The drawing under review shows one solid part. Ordinate dimensions are in mm from its lowest x, y, z. Coordinates: 2 decimals unless noted, no trailing zeros. Write each loop counter-clockwise with the first axis right and the second up, starting at its lowest first coordinate (ties: lowest second). Pieces come first, ordered by that corner, then holes. Notation, with made-up numbers: M 83.25,30.5 L 106.25,30.5 A17 ccw 106.25,50.5 Z; hole C 32,-5 d2. An arc over 180 degrees is marked long. Write each question's results on one line, items separated by ' | '. Start each with the question number.
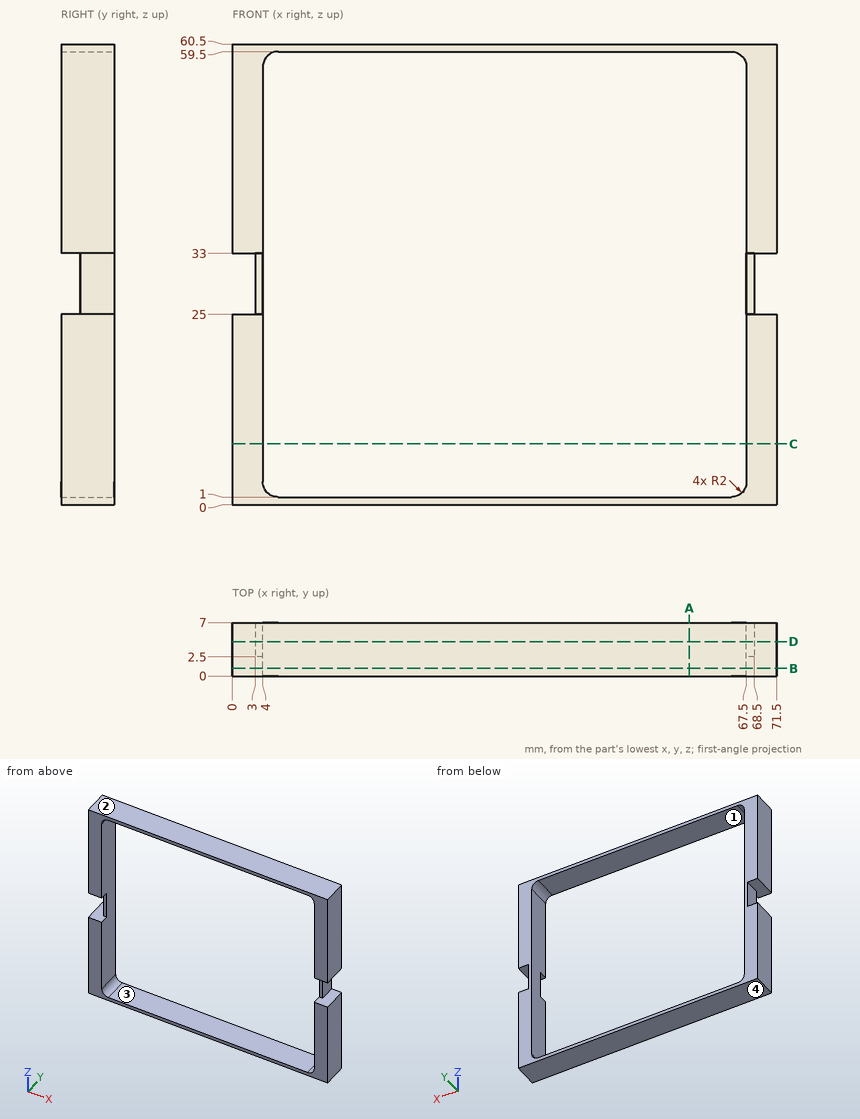
Item 1: We need section C-C on z = 8. State the section outline as (x, y) points, then the cut area to 3 significant figures.
Item 2: Wall thickness on L1, parallel to Z at x = 27, y = 4.25; L2, parallel to X at y = 1, z = 15; L3, parallel to X at y = 4.5, z = 26.5: over which ranges is each line inside the solid? List them lowest first.
Item 3: Draft analysis for pull direction Z (two halves, no side actions). For the marked faces 1, 2, 3 and 4, state which applies: released by +Z, released by -Z, zero draft, split by the parting line, or undercut.
Item 4: We need section B-B on y = 1. State the section outline as (x, z) points.
Item 5: We need section D-D on y = 4.5. State the section outline as (x, z) points, then the cut area to 3 significant figures.
Item 6: Insertion check: pin 1 Ø1 at (x, y) = (45.5, 1.5) entering from -Z; pin 2 Ø3.5 at (y, z) = (4, 29.5) entering from +X; pin 3 Ø0.5 at (x, z) = (3.5, 30.5) entering from -Y; pin 4 Ø3.5 at (y, z) = (4, 29.5) entering from -X. Each pin has a flat end and moves straight along its axis. Give the tip position at first contact, or say it passes through.
Item 7: We need section A-A on x = 60. State the section outline as (y, z) points.
Answer:
1) outline: M 0,0 L 4,0 L 4,7 L 0,7 Z; M 67.5,0 L 71.5,0 L 71.5,7 L 67.5,7 Z | area: 56.0 mm^2
2) L1: z = 0 to 1, 59.5 to 60.5 | L2: x = 0 to 4, 67.5 to 71.5 | L3: x = 3 to 4, 67.5 to 68.5
3) face 1: undercut | face 2: released by +Z | face 3: undercut | face 4: released by -Z
4) outline: M 0,0 L 71.5,0 L 71.5,25 L 67.5,25 L 67.5,3 A2 cw 65.5,1 L 6,1 A2 cw 4,3 L 4,25 L 0,25 Z; M 0,33 L 4,33 L 4,57.5 A2 cw 6,59.5 L 65.5,59.5 A2 cw 67.5,57.5 L 67.5,33 L 71.5,33 L 71.5,60.5 L 0,60.5 Z
5) outline: M 0,0 L 71.5,0 L 71.5,25 L 68.5,25 L 68.5,33 L 71.5,33 L 71.5,60.5 L 0,60.5 L 0,33 L 3,33 L 3,25 L 0,25 Z; hole M 4,3 A2 ccw 6,1 L 65.5,1 A2 ccw 67.5,3 L 67.5,57.5 A2 ccw 65.5,59.5 L 6,59.5 A2 ccw 4,57.5 Z | area: 566 mm^2
6) pin 1: stops at z = 0 | pin 2: stops at x = 68.5 | pin 3: stops at y = 2.5 | pin 4: stops at x = 3
7) outline: M 0,0 L 7,0 L 7,1 L 0,1 Z; M 0,59.5 L 7,59.5 L 7,60.5 L 0,60.5 Z
